Source: CAD feature listing. Evaluate the final solid. Frame: model axes, mm. Give positions to 0.01 mm unless a question says otherwise; leave off trailing zeros. Loops run counter-clockwise (first coordinate to the right, second up) from the corner with the lowest first, then second, coordinate; pieces in that order, holes last. Notation, with made-up numbers: M 26,-24 L 72,-24 A21 cw 72,3 Z; hole C 9.5,42 d3. An arc over 180 degrees is marked long. Answer in a Markdown table with one row per item.
```python
from build123d import *

# Parameters (mm, degrees)
F0_R     = 3.5
F1_DEPTH = 1


with BuildPart() as f1:
    # F0 (on Front) → F1 (new body)
    with BuildSketch(Plane.XZ):
        with BuildLine():
            Line((-6.6117709503, -17.7072025836), (-4.180541262, -15.3958080336))
            Line((-4.180541262, -15.3958080336), (-4.0357941762, -9.6612172201))
            ThreePointArc((-4.0357941762, -9.6612172201), (-0.8592229863, -7.0206183808), (2.2847101224, -9.6999935621))
            Line((2.2847101224, -9.6999935621), (2.2847101224, -14.6249644458))
            Line((2.2847101224, -14.6249644458), (3.3562604804, -16.0533804446))
            Line((3.3562604804, -16.0533804446), (4.2133103125, -16.0533804446))
            Line((4.2133103125, -16.0533804446), (5.123925861, -14.5599710971))
            Line((5.123925861, -14.5599710971), (5.123925861, -12.2859868333))
            ThreePointArc((5.123925861, -12.2859868333), (4.9774792516, -11.9324334427), (4.623925861, -11.7859868333))
            Line((4.623925861, -11.7859868333), (3.6633914474, -11.7859868333))
            ThreePointArc((3.6633914474, -11.7859868333), (3.5219700912, -11.7274081895), (3.4633914474, -11.5859868333))
            Line((3.4633914474, -11.5859868333), (3.4633914474, -9.3933893368))
            ThreePointArc((3.4633914474, -9.3933893368), (3.6098380568, -9.0398359462), (3.9633914474, -8.8933893368))
            Line((3.9633914474, -8.8933893368), (6.0659102777, -8.8933893368))
            ThreePointArc((6.0659102777, -8.8933893368), (6.4194636683, -8.7469427274), (6.5659102777, -8.3933893368))
            Line((6.5659102777, -8.3933893368), (6.5659102777, -7.6971449889))
            add(Edge.make_bspline(
                [(6.5659102777, -7.6971449889), (6.5659102777, -7.3604537174), (6.1308538816, -6.7250376157), (5.3694360763, -5.3256448251), (5.0200880103, -3.2005265741), (5.1779062539, -1.5597114412), (5.5472315899, -0.5191652161), (5.7321804401, 0)],
                knots=[0, 0, 0, 0, 0.1603623278, 0.3613989356, 0.5935239119, 0.7972784215, 1, 1, 1, 1], degree=3))
            ThreePointArc((5.7321804401, 0), (-1.0752950501, 9.7383416681), (-6.8182754475, -0.663350365))
            add(Edge.make_bspline(
                [(-7.9565616325, -9.7683481872), (-7.8795153177, -9.2354358822), (-7.7383664617, -8.0850617885), (-6.3860842213, -6.2946925646), (-6.072886576, -4.0949884517), (-6.0697572799, -2.3374053261), (-6.5696365594, -1.2250004752), (-6.8182754475, -0.663350365)],
                knots=[0, 0, 0, 0, 0.1859272011, 0.4003477057, 0.6149796646, 0.8054836062, 1, 1, 1, 1], degree=3))
            Line((-7.9565616325, -9.7683481872), (-7.9565616325, -11.7456736863))
            ThreePointArc((-7.9565616325, -11.7456736863), (-7.810115023, -12.0992270769), (-7.4565616325, -12.2456736863))
            Line((-7.4565616325, -12.2456736863), (-7.3690715705, -12.2456736863))
            ThreePointArc((-7.3690715705, -12.2456736863), (-7.0135065314, -12.3941434558), (-6.8691041299, -12.7513796745))
            Line((-6.8691041299, -12.7513796745), (-6.9242371246, -17.5822172314))
            ThreePointArc((-6.9242371246, -17.5822172314), (-6.8108358449, -17.7517903835), (-6.6117709503, -17.7072025836))
        make_face()
        with Locations((-0.7007342175, 2.7600016318)):
            Circle(F0_R, mode=Mode.SUBTRACT)
    extrude(amount=F1_DEPTH)


solid = f1.part
```
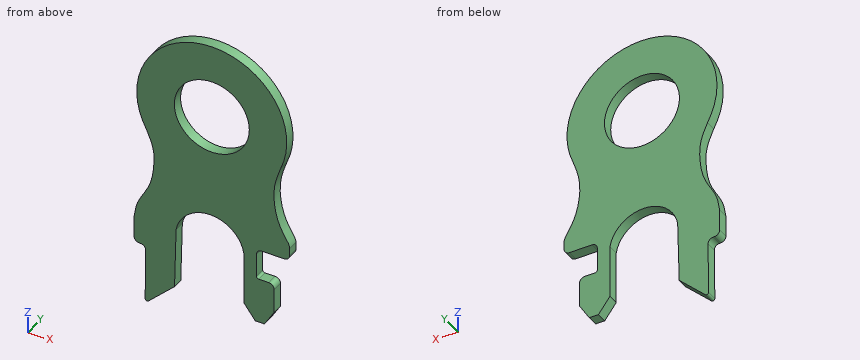
Q1. Section query C-C (x = -4.75). Output: boundary loops of the cut face in (y, z).
Values follow:
| item | result |
|---|---|
| outline | M -1,-15.94 L 0,-15.94 L 0,8.46 L -1,8.46 Z |
Q2. Ray query, probe 1 along Z at (x, y) = (-1.25, -0.55); probe 2 along X at (y, z) = (-0.4, 0.25); probe 3 along X at (y, z) = (-0.5, -8.5). Return the intervals inside material, ascending. Write a range as from..to.
Values follow:
| item | result |
|---|---|
| probe 1 | -7.04..-0.7, 6.22..9.73 |
| probe 2 | -7.24..-3.14, 1.74..5.83 |
| probe 3 | -7.71..-3.58, 1.82..6.55 |
Q3. Section query A-A (x = 1). Output: boundary loops of the cut face in (y, z).
Values follow:
| item | result |
|---|---|
| outline | M -1,-7.63 L 0,-7.63 L 0,-0.3 L -1,-0.3 Z; M -1,5.82 L 0,5.82 L 0,9.54 L -1,9.54 Z |
Q4. Section query B-B (z = -14). Output: boundary loops of the cut face in (x, y).
Values follow:
| item | result |
|---|---|
| outline | M -6.88,-1 L -4.15,-1 L -4.15,0 L -6.88,0 Z; M 2.28,-1 L 5.12,-1 L 5.12,0 L 2.28,0 Z |
Q5. Contact query for flat-ended pins moving along their axis: pin 1 Ø0.5 at (y, z) = (-0.5, -13) entering from -X; pin 2 Ø6.5 at (x, z) = (-0.7, 2.76) entering from +Y; pin 3 Ø0.5 at (y, z) = (-0.5, -10.5) entering from +X. Output: stop coordinate, or through.
Values follow:
| item | result |
|---|---|
| pin 1 | x = -6.87 |
| pin 2 | through |
| pin 3 | x = 3.46 |
